Part model, mm, in its own coordinate system. Face numbers are marked on the shaded views. A direction names the side the tool comes from. Coordinates: 2 decimals unless noted, no trailing zeros. Write each loop counter-clockwise with the first axis right and the second up, starting at its lowest first coordinate (ties: lowest second). Pieces come first, ordered by that corner, then holes. Notation, with made-up numbers: (-37, 87) - (4, 87) arc R16 ccw to (4, 113) - close; hole circle Ø8 at (61, 71). An arc over 180 degrees is marked (long way). Use a Markdown table: item, result.
Autodesk Inventor part; units mm, degrees
ref_plane "YZ Plane" through (0, 0, 0) normal (1, 0, 0) x (0, 1, 0)
ref_plane "XZ Plane" through (0, 0, 0) normal (0, 1, 0) x (-1, 0, 0)
ref_plane "XY Plane" through (0, 0, 0) normal (0, 0, 1) x (1, 0, 0)
sketch "Sketch1" plane through (0, 0, 0) normal (0, 1, 0) x (-1, 0, 0)
  line L0 (-52.5, 27.5) -> (52.5, 27.5)
  line L1 (52.5, 27.5) -> (52.5, -27.5)
  line L2 (52.5, -27.5) -> (-52.5, -27.5)
  line L3 (-52.5, -27.5) -> (-52.5, 27.5)
  line L4 (-52.5, 27.5) -> (52.5, -27.5) construction
  line L5 (52.5, 27.5) -> (-52.5, -27.5) construction
  line L6 (52.5, 19.5) -> (44.5, 27.5)
  line L7 (52.5, -19.5) -> (44.5, -27.5)
  line L8 (-44.5, 27.5) -> (-52.5, 19.5)
  line L9 (-52.5, -19.5) -> (-44.5, -27.5)
  point P0 (0, 0)
  dimension "d0" = 105
  dimension "d1" = 55
  dimension "d4" = 45
  dimension "d5" = 8
  dimension "d6" = 8
  dimension "d7" = 8
  dimension "d8" = 8
extrude "Extrusion1" add sketch "Sketch1" along normal blind 25 contours L0 L6 L1 L7 L2 L9 L3 L8
shell "Shell1" thickness 3 outward yes removed faces 1 at (-14.8333, 25, -9.1667)
sketch "Sketch2" plane through (0, 25, 0) normal (0, 1, 0) x (1, 0, 0)
  line L0 (-55.5, 20.7426) -> (-55.5, -20.7426)
  line L1 (-52.5, -19.5) -> (-52.5, 19.5)
  line L2 (-55.5, 7.5) -> (-52.5, 7.5)
  line L3 (-52.5, 7.5) -> (-52.5, -7.5)
  line L4 (-52.5, -7.5) -> (-55.5, -7.5)
  line L5 (-55.5, -7.5) -> (-55.5, 7.5)
  line L6 (55.5, -20.7426) -> (55.5, 20.7426)
  line L7 (52.5, 7.5) -> (55.5, 7.5)
  line L8 (55.5, 7.5) -> (55.5, -7.5)
  line L9 (55.5, -7.5) -> (52.5, -7.5)
  line L10 (52.5, -7.5) -> (52.5, 7.5)
  line L11 (52.5, 19.5) -> (52.5, -19.5)
  point P0 (0, 0)
  point P1 (-54, -7.5)
  point P2 (-52.5, 0)
  point P3 (-52.5, 0)
  point P4 (54, -7.5)
  point P5 (54, 7.5)
  point P6 (52.5, 0)
  point P7 (52.5, 0)
  dimension "d10" = 15
  dimension "d11" = 0
  dimension "d12" = 0
  dimension "d13" = 15
  dimension "d14" = 0
extrude "Extrusion2" cut sketch "Sketch2" against normal blind 15
properties part number "case_v1"
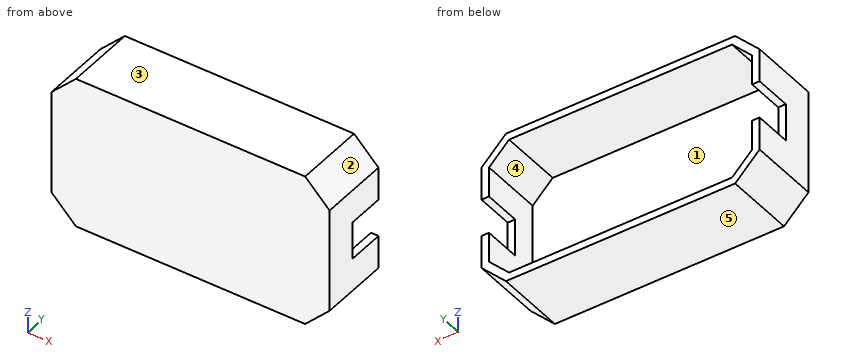
Item 1: Band-saw the part on A-A, the plane y = 16.75. Give the cut face in (x, z).
From the geometry:
| item | result |
|---|---|
| outline | (-55.5, -20.74) - (-45.74, -30.5) - (45.74, -30.5) - (55.5, -20.74) - (55.5, -7.5) - (52.5, -7.5) - (52.5, -19.5) - (44.5, -27.5) - (-44.5, -27.5) - (-52.5, -19.5) - (-52.5, -7.5) - (-55.5, -7.5) - close; (-55.5, 7.5) - (-52.5, 7.5) - (-52.5, 19.5) - (-44.5, 27.5) - (44.5, 27.5) - (52.5, 19.5) - (52.5, 7.5) - (55.5, 7.5) - (55.5, 20.74) - (45.74, 30.5) - (-45.74, 30.5) - (-55.5, 20.74) - close |
Item 2: Band-saw the part on C-C, the plane y = 6.75. Give the cut face in (x, z), then the cut area to 3 significant figures.
From the geometry:
| item | result |
|---|---|
| outline | (-55.5, -20.74) - (-45.74, -30.5) - (45.74, -30.5) - (55.5, -20.74) - (55.5, 20.74) - (45.74, 30.5) - (-45.74, 30.5) - (-55.5, 20.74) - close; hole (-52.5, -19.5) - (-44.5, -27.5) - (44.5, -27.5) - (52.5, -19.5) - (52.5, 19.5) - (44.5, 27.5) - (-44.5, 27.5) - (-52.5, 19.5) - close |
| area | 934 mm^2 |
Item 3: Two-plate mould, pull along X, no slides. Class the marked faces 1, 2 and 3: pulls with the +X half, pulls with the -X half, needs draft (parallel to the pull), parting line crosses it, or undercut.
From the geometry:
| item | result |
|---|---|
| face 1 | undercut |
| face 2 | pulls with the +X half |
| face 3 | needs draft |
Item 4: Band-saw the part on D-D, the plane x = 38.5. Give the cut face in (y, z), then the cut area to 3 significant figures.
From the geometry:
| item | result |
|---|---|
| outline | (-3, -30.5) - (25, -30.5) - (25, -27.5) - (0, -27.5) - (0, 27.5) - (25, 27.5) - (25, 30.5) - (-3, 30.5) - close |
| area | 333 mm^2 |
Item 5: Band-saw the part on B-B, the plane z = -16. Give the cut face in (x, y), then the cut area to 3 significant figures.
From the geometry:
| item | result |
|---|---|
| outline | (-55.5, -3) - (55.5, -3) - (55.5, 25) - (52.5, 25) - (52.5, 0) - (-52.5, 0) - (-52.5, 25) - (-55.5, 25) - close |
| area | 483 mm^2 |
Item 6: Drill centre lines: probe 1 along Z at (x, y) = (38, 16); probe 2 along X at (y, z) = (23.75, -15); probe 3 along Y at (x, z) = (-8, 23.5). Where is each one in solid material? Low to high.
From the geometry:
| item | result |
|---|---|
| probe 1 | -30.5 to -27.5, 27.5 to 30.5 |
| probe 2 | -55.5 to -52.5, 52.5 to 55.5 |
| probe 3 | -3 to 0 |
Item 7: Drop flat-ended pins along their axis: P1, Ø2.5, axis at x = -54.5, y = 20.5, coming from the +Z side; P2, Ø1.5, axis at x = 11.5, z = 19.5, coming from the +Y side; P3, Ø0.9, axis at x = 54.5, z = -3, coming from the +Y side. Give the stop position or say it passes through.
From the geometry:
| item | result |
|---|---|
| P1 | z = 22.99 |
| P2 | y = 0 |
| P3 | y = 10 |
Item 8: Which spindle directions (+Z, -Z, +X, -X, +Y, -Y) get a long thin tool onto all of the face, cutting with end or side? Do the marked faces 4 and 5. Say none if no direction does.
From the geometry:
| item | result |
|---|---|
| face 4 | +Y |
| face 5 | -Z, +X, -X, +Y, -Y |
